Could you check a few things on this model? Use its own coordinates, in mm. Face numbers are marked on the shaded views. A direction names the side the tool comes from. Give positions to 0.01 mm unless a question says otherwise; leave off trailing zeros. Loops run counter-clockwise (first coordinate to the right, second up) from the corner with the lowest first, then second, coordinate; pieces in that order, holes last. Notation, with made-up numbers: M 55,1.25 L 103,1.25 A13 cw 103,26.25 Z; hole C -6.75,74 d10. An arc over 180 degrees is marked long. Use a Markdown table: item, result. Add a question column.
1) If I drill on line 1 along Y through (x, z) = (-29, 2.5); line 2 along Z through (x, y) = (-19.5, 23); line 3 along Y through (x, z) = (8, 1), over which ranges is the centre line in solid material (lowest first)? Write a range as [from, to].
2) Suppose I cut it at C-C on y = -12.5. List the corners of the cut face in (x, z) for me.
3) Suppose I cut it at D-D on y = 22.5. List the corners of the cut face in (x, z) for me, and give its area (3 significant figures).
4) Suppose I cut it at B-B on x = -5. List the corners of the cut face in (y, z) for me.
5) Suppose I cut it at A-A on z = 4.25. List the corners of the cut face in (x, y) for me.
6) Which directions (+Z, -Z, +X, -X, +Y, -Y) give clear straight access to the entire face, cutting with the end or side of a thin tool? Please do the marked faces 1 and 2.
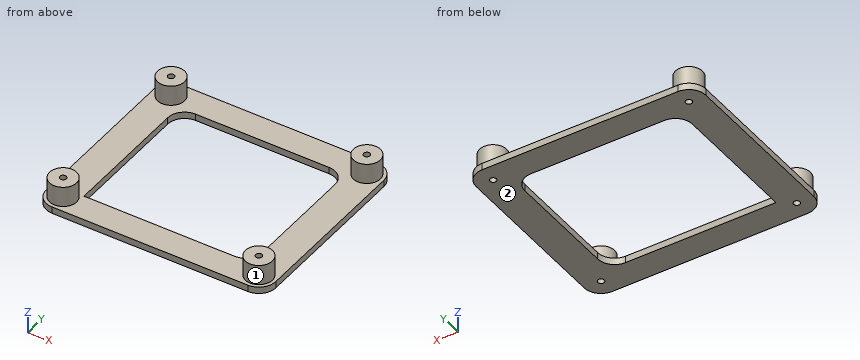
```python
from build123d import *

# Parameters (mm, degrees)
SKETCH1_W           = 68
SKETCH1_H           = 59
SKETCH1_R           = 0.95
SKETCH1_W_2         = 49.559322034
SKETCH1_H_2         = 43
BOSS_EXTRUDE1_DEPTH = 2
SKETCH2_R           = 4
SKETCH2_R_2         = 0.95
BOSS_EXTRUDE2_DEPTH = 6
FILLET1_R           = 5


with BuildPart() as part:
    # Sketch1 → Boss-Extrude1 (new body)
    with BuildSketch(Plane.XY):
        Rectangle(SKETCH1_W, SKETCH1_H)
        with Locations((-29, 24.5)):
            Circle(SKETCH1_R, mode=Mode.SUBTRACT)
        with Locations((29, 24.5)):
            Circle(SKETCH1_R, mode=Mode.SUBTRACT)
        with Locations((29, -24.5)):
            Circle(SKETCH1_R, mode=Mode.SUBTRACT)
        with Locations((-29, -24.5)):
            Circle(SKETCH1_R, mode=Mode.SUBTRACT)
        Rectangle(SKETCH1_W_2, SKETCH1_H_2, mode=Mode.SUBTRACT)
    extrude(amount=BOSS_EXTRUDE1_DEPTH)

    # Sketch2 → Boss-Extrude2 (add)
    # profile 1 of 4: a face of its own
    with BuildSketch(Plane.XY.offset(2)):
        with Locations(Location((-29, 24.5, 0), (0, 0, 180))):
            Circle(SKETCH2_R)
        with Locations((-29, 24.5)):
            Circle(SKETCH2_R_2, mode=Mode.SUBTRACT)
    # profile 2 of 4: a face of its own
    with BuildSketch(Plane.XY.offset(2)):
        with Locations(Location((29, 24.5, 0), (0, 0, 180))):
            Circle(SKETCH2_R)
        with Locations((29, 24.5)):
            Circle(SKETCH2_R_2, mode=Mode.SUBTRACT)
    # profile 3 of 4: a face of its own
    with BuildSketch(Plane.XY.offset(2)):
        with Locations(Location((29, -24.5, 0), (0, 0, 180))):
            Circle(SKETCH2_R)
        with Locations((29, -24.5)):
            Circle(SKETCH2_R_2, mode=Mode.SUBTRACT)
    # profile 4 of 4: a face of its own
    with BuildSketch(Plane.XY.offset(2)):
        with Locations(Location((-29, -24.5, 0), (0, 0, 180))):
            Circle(SKETCH2_R)
        with Locations((-29, -24.5)):
            Circle(SKETCH2_R_2, mode=Mode.SUBTRACT)
    extrude(amount=BOSS_EXTRUDE2_DEPTH)

    # Fillet1
    fillet1_edges = [part.edges().sort_by_distance(p)[0] for p in [
        (24.779661017, -21.5, 1),
        (24.779661017, 21.5, 1),
        (-24.779661017, 21.5, 1),
        (34, -29.5, 1),
        (-34, -29.5, 1),
        (-34, 29.5, 1),
        (34, 29.5, 1),
    ]]
    fillet(fillet1_edges, radius=FILLET1_R)


solid = part.part
```
Answer block:
| question | item | result |
|---|---|---|
| 1 | line 1 | y = [-28.5, -25.45], [-23.55, -20.5], [20.5, 23.55], [25.45, 28.5] |
| 1 | line 2 | z = [0, 2] |
| 1 | line 3 | y = [-29.5, -21.5], [21.5, 29.5] |
| 2 | outline | M -34,0 L -24.78,0 L -24.78,2 L -34,2 Z; M 24.78,0 L 34,0 L 34,2 L 24.78,2 Z |
| 3 | outline | M -34,0 L 34,0 L 34,2 L 32.46,2 L 32.46,8 L 25.54,8 L 25.54,2 L -25.54,2 L -25.54,8 L -32.46,8 L -32.46,2 L -34,2 Z |
| 3 | area | 219 mm^2 |
| 4 | outline | M -29.5,0 L -21.5,0 L -21.5,2 L -29.5,2 Z; M 21.5,0 L 29.5,0 L 29.5,2 L 21.5,2 Z |
| 5 | outline | C -29,-24.5 d8; C -29,24.5 d8; C 29,-24.5 d8; C 29,24.5 d8; hole C -29,-24.5 d1.9; hole C -29,24.5 d1.9; hole C 29,-24.5 d1.9; hole C 29,24.5 d1.9 |
| 6 | face 1 | +Z |
| 6 | face 2 | -Z, +X, -X, +Y, -Y |
